```python
from build123d import *

# Parameters (mm, degrees)
F0_W     = 63.5
F0_H     = 63.499996
F1_DEPTH = 3.81
F2_R     = 11.5062
F3_DEPTH = 12.7
F4_R     = 9.525
F5_DEPTH = 0.9906


with BuildPart() as f1:
    # F0 (on Top) → F1 (new body)
    with BuildSketch(Plane.XY):
        Rectangle(F0_W, F0_H)
    extrude(amount=F1_DEPTH)

    # F2 (on face) → F3 (join)
    with BuildSketch(Plane.XY.offset(3.81)):
        Circle(F2_R)
    extrude(amount=F3_DEPTH)

    # F4 (on face) → F5 (cut)
    with BuildSketch(Plane.XY.offset(16.51)):
        Circle(F4_R)
    extrude(amount=-F5_DEPTH, mode=Mode.SUBTRACT)


solid = f1.part
```
Check sheet for the modelled part. Datum: model origin and axes. Units: mm. A direction names the side the tool comes from. Coordinates: 2 decimals unless noted, no trailing zeros. Loops run counter-clockwise (first coordinate to the right, second up) from the corner with the lowest first, then second, coordinate; pieces in that order, holes last.
1) Sectioned sample at C-C (z = 11). Record the boundary of the cut face in (x, y).
2) Access from +Z, -Z, +X, -X, +Y, -Y to the whole of each face (thin tool, end or side, straight path). Record for faces 1 (the face through (-7.559, -5.796, 16.022)), 2 (the face through (31.75, 0, 2)).
3) Material ranges on probe 1 along Y at (x, z) = (0, 16.1) (3 decimals); probe 2 along Z at (x, y) = (-16, 15); probe 3 along X at (y, z) = (-6.5, 5.25), recorded low to high.
4) Sectioned sample at D-D (y = 27.5). Record the boundary of the cut face in (x, z), and give its area (3 significant figures).
5) Release check for a two-part mould opening along Y. For faces 3 (the face through (-2.494, -11.233, 10.071)), 4 (the face through (0, 15, 3.81)), 5 (the face through (0, 0, 15.519)) record: released by +Y, released by -Y, zero draft, split by the parting line, or undercut.
6) Sectioned sample at A-A (y = 0). Record the boundary of the cut face in (x, z) (3 decimals).
7) Gauge pin test, flat ends, axial feed: pin 1 (4 mm diameter, centred on x = -5.5, y = 21.5, fed in from +Z); pin 2 (3 mm diameter, centred on y = -9, z = 7, fed in from -X). Record the tip position at first contact, or that the pin passes through.
8) Sectioned sample at B-B (x = 6). Record the boundary of the cut face in (y, z).
Check sheet entries:
1. outline: circle Ø23.01 at (0, 0)
2. face 1: +Z
2. face 2: +Z, -Z, +X, +Y, -Y
3. probe 1: y = -11.506 to -9.525, 9.525 to 11.506
3. probe 2: z = 0 to 3.81
3. probe 3: x = -9.49 to 9.49
4. outline: (-31.75, 0) - (31.75, 0) - (31.75, 3.81) - (-31.75, 3.81) - close
4. area: 242 mm2
5. face 3: split by the parting line
5. face 4: zero draft
5. face 5: undercut
6. outline: (-31.75, 0) - (31.75, 0) - (31.75, 3.81) - (11.506, 3.81) - (11.506, 16.51) - (9.525, 16.51) - (9.525, 15.519) - (-9.525, 15.519) - (-9.525, 16.51) - (-11.506, 16.51) - (-11.506, 3.81) - (-31.75, 3.81) - close
7. pin 1: stops at z = 3.81
7. pin 2: stops at x = -8.73
8. outline: (-31.75, 0) - (31.75, 0) - (31.75, 3.81) - (9.82, 3.81) - (9.82, 16.51) - (7.4, 16.51) - (7.4, 15.52) - (-7.4, 15.52) - (-7.4, 16.51) - (-9.82, 16.51) - (-9.82, 3.81) - (-31.75, 3.81) - close
